```python
from build123d import *

# Parameters (mm, degrees)
F0_W      = 30
F0_H      = 30
F1_DEPTH  = 30
F5_R      = 1.25
F7_W      = 25
F7_H      = 25
F8_DEPTH  = 30
F9_W      = 29.9418475479
F9_H      = 30.1353819668
F10_DEPTH = 5


with BuildPart() as f1:
    # F0 (on Top) → F1 (new body)
    with BuildSketch(Plane.XY):
        with Locations((15, 15)):
            Rectangle(F0_W, F0_H)
    extrude(amount=F1_DEPTH)

    # F6: sweep along a path in F4
    with BuildLine(Plane(origin=(0, 15, 0), x_dir=(-1, 0, 0), z_dir=(0, 1, 0))) as f6_path:
        ThreePointArc((-27, 30), (-25.5355339059, 33.5355339059), (-22, 35))
        Line((-22, 35), (-8, 35))
        ThreePointArc((-8, 35), (-4.4644660941, 33.5355339059), (-3, 30))
    # F5 (on face) → F6 (sweep)
    with BuildSketch(Plane.XY.offset(30)):
        with Locations((26.8965084106, 14.8129407316)):
            Circle(F5_R)
    sweep(path=f6_path.line)

    # F7 (on face) → F8 (cut, through all)
    with BuildSketch(Plane(origin=(0, 0, 0), x_dir=(1, 0, 0), z_dir=(0, 0, -1))):
        with Locations((15, -15)):
            Rectangle(F7_W, F7_H)
    extrude(amount=-F8_DEPTH, mode=Mode.SUBTRACT)

    # F9 (on face) → F10 (join)
    with BuildSketch(Plane.XY.offset(30)):
        with Locations((14.9709237739, 15.0676909834)):
            Rectangle(F9_W, F9_H)
    extrude(amount=-F10_DEPTH)


solid = f1.part
```
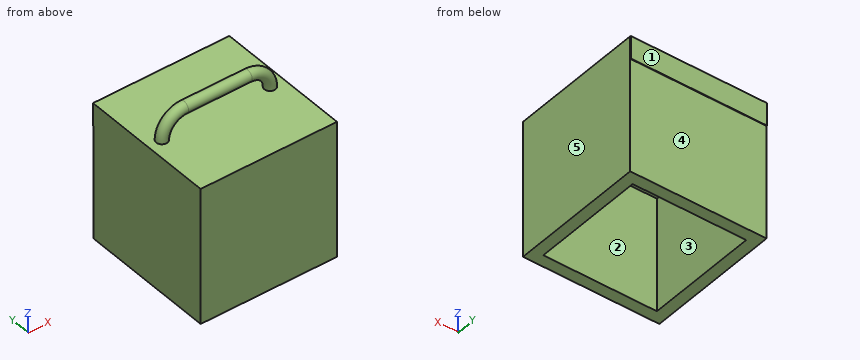
Source: CAD feature listing. Evaluate the final solid. Frame: model axes, mm. Face numbers are marked on the shaded views. A direction names the side the tool comes from. Coordinates: 2 decimals unless noted, no trailing zeros. Loops run counter-clockwise (first coordinate to the right, second up) from the corner with the lowest first, then second, coordinate; pieces in that order, holes last. Notation, with made-up numbers: M 38.5,45.5 L 63.5,45.5 A35 cw 63.5,80.5 Z; hole C 6.25,42 d1. An arc over 180 degrees is marked long. Use a Markdown table: item, result. Add a question column.
Q1. Section query A-A, the plane x = 19.5. Return loops of the section in (y, z).
Q2. Section query C-C, the plane y = 24.5. Return loops of the section in (x, z), and give its area (3 significant figures).
Q3. Material intervals for L1, parallel to Y at x = 18, z = 6; L2, parallel to Z at x = 13, y = 25.5, sorted ascending.
Q4. Access query for the marked faces 1 and 2. Directions: +Z, -Z, +X, -X, +Y, -Y. A direction counts if a zero-diameter tool reaches every point of the face in a straight line with its end or side. Return the directions, or none.
Q5. Section query B-B, the plane z = 13.5. Return loops of the section in (x, y).
Q6. First-contact query: pin 1 (6 mm diameter, centred on x = 9.5, y = 25, fed in from +Z); pin 2 (2 mm diameter, centred on x = 25, z = 32.5, fed in from +Y); pin 3 (8 mm diameter, centred on x = 11, z = 14, fed in from +Y). Flat tips, straight axial feed; report the tip coordinate or a pass-through.
Q7. Draft query along X for the marked faces 3, 4 and 5. Return one class per face: pulls with the +X half, pulls with the -X half, needs draft (parallel to the pull), parting line crosses it, or undercut.
Result:
| question | item | result |
|---|---|---|
| 1 | outline | M 0,0 L 2.5,0 L 2.5,25 L 27.5,25 L 27.5,0 L 30,0 L 30,25 L 30.14,25 L 30.14,30 L 0,30 Z; C 14.81,34.9 d2.5 |
| 2 | outline | M 0,0 L 2.5,0 L 2.5,25 L 27.5,25 L 27.5,0 L 30,0 L 30,30 L 0,30 Z |
| 2 | area | 275 mm2 |
| 3 | L1 | y = 0 to 2.5, 27.5 to 30 |
| 3 | L2 | z = 25 to 30 |
| 4 | face 1 | +Z, -Z, +X, -X, +Y |
| 4 | face 2 | -Z |
| 5 | outline | M 0,0 L 30,0 L 30,30 L 0,30 Z; hole M 2.5,2.5 L 27.5,2.5 L 27.5,27.5 L 2.5,27.5 Z |
| 6 | pin 1 | stops at z = 30 |
| 6 | pin 2 | stops at y = 16.06 |
| 6 | pin 3 | stops at y = 30 |
| 7 | face 3 | undercut |
| 7 | face 4 | needs draft |
| 7 | face 5 | pulls with the +X half |
